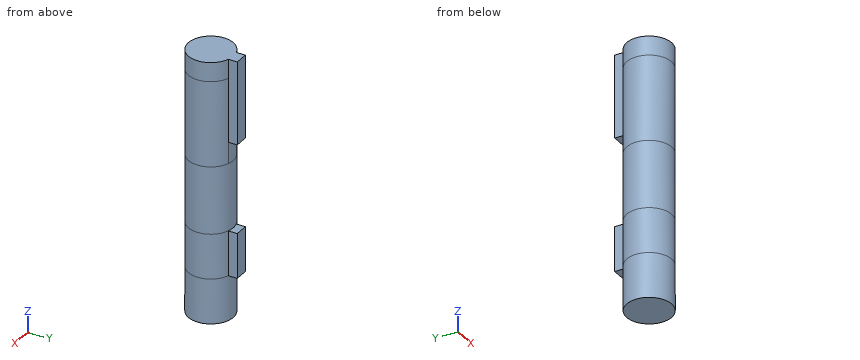
from build123d import *

# Parameters (mm, degrees)
SKETCH1_R            = 5
BOSS_EXTRUDE1_DEPTH  = 20
BOSS_EXTRUDE2_DEPTH  = 10
SKETCH4_R            = 5
BOSS_EXTRUDE3_DEPTH  = 27
BOSS_EXTRUDE4_DEPTH  = 19
SKETCH6_R            = 5
BOSS_EXTRUDE5_DEPTH  = 30
SKETCH7_R            = 5
CUT_EXTRUDE1_DEPTH   = 10
SKETCH8_R            = 6.933887
CUT_EXTRUDE2_DEPTH   = 35
SKETCH9_R            = 5
CUT_EXTRUDE3_DEPTH   = 12
SKETCH10_R           = 5
BOSS_EXTRUDE8_DEPTH  = 15
BOSS_EXTRUDE9_DEPTH  = 10
SKETCH12_R           = 5
BOSS_EXTRUDE10_DEPTH = 10
SKETCH13_R           = 5
CUT_EXTRUDE4_DEPTH   = 28
SKETCH20_R           = 5
CUT_EXTRUDE5_DEPTH   = 2
BOSS_EXTRUDE11_DEPTH = 4.25
CUT_EXTRUDE6_DEPTH   = 22.25
BOSS_EXTRUDE12_DEPTH = 17.5


with BuildPart() as part:
    # Sketch1 → Boss-Extrude1 (new body)
    with BuildSketch(Plane.XY):
        Circle(SKETCH1_R)
    extrude(amount=BOSS_EXTRUDE1_DEPTH)

    # Sketch3 → Boss-Extrude2 (add)
    with BuildSketch(Plane.XY.offset(20)):
        with BuildLine():
            Line((1.5, 6.769696), (-1.5, 6.769696))
            Line((-1.5, 6.769696), (-1.5, 4.769696))
            ThreePointArc((-1.5, 4.769696), (0, -5), (1.5, 4.769696))
            Line((1.5, 4.769696), (1.5, 6.769696))
        make_face()
    extrude(amount=BOSS_EXTRUDE2_DEPTH)

    # Sketch4 → Boss-Extrude3 (add)
    with BuildSketch(Plane.XY.offset(30)):
        Circle(SKETCH4_R)
    extrude(amount=BOSS_EXTRUDE3_DEPTH)

    # Sketch5 → Boss-Extrude4 (add)
    with BuildSketch(Plane.XY.offset(57)):
        with BuildLine():
            Line((-1.5, 4.769696), (-1.5, 6.769696))
            Line((-1.5, 6.769696), (1.5, 6.769696))
            Line((1.5, 6.769696), (1.5, 4.769696))
            ThreePointArc((1.5, 4.769696), (0, -5), (-1.5, 4.769696))
        make_face()
    extrude(amount=BOSS_EXTRUDE4_DEPTH)

    # Sketch6 → Boss-Extrude5 (add)
    with BuildSketch(Plane.XY.offset(76)):
        Circle(SKETCH6_R)
    extrude(amount=BOSS_EXTRUDE5_DEPTH)

    # Sketch7 → Cut-Extrude1 (cut)
    with BuildSketch(Plane(origin=(0, 0, 0), x_dir=(-1, 0, 0), z_dir=(0, 0, -1))):
        Circle(SKETCH7_R)
    extrude(amount=-CUT_EXTRUDE1_DEPTH, mode=Mode.SUBTRACT)

    # Sketch8 → Cut-Extrude2 (cut)
    with BuildSketch(Plane(origin=(0, 0, 10), x_dir=(-1, 0, 0), z_dir=(0, 0, -1))):
        Circle(SKETCH8_R)
    extrude(amount=-CUT_EXTRUDE2_DEPTH, mode=Mode.SUBTRACT)

    # Sketch9 → Cut-Extrude3 (cut)
    with BuildSketch(Plane(origin=(0, 0, 45), x_dir=(-1, 0, 0), z_dir=(0, 0, -1))):
        with Locations(Location((0, 0, 0), (0, 0, 72.542397))):
            Circle(SKETCH9_R)
    extrude(amount=-CUT_EXTRUDE3_DEPTH, mode=Mode.SUBTRACT)

    # Sketch10 → Boss-Extrude8 (add)
    with BuildSketch(Plane(origin=(0, 0, 57), x_dir=(-1, 0, 0), z_dir=(0, 0, -1))):
        Circle(SKETCH10_R)
    extrude(amount=BOSS_EXTRUDE8_DEPTH)

    # Sketch11 → Boss-Extrude9 (add)
    with BuildSketch(Plane(origin=(0, 0, 42), x_dir=(-1, 0, 0), z_dir=(0, 0, -1))):
        with BuildLine():
            Line((-1.5, 6.769696), (1.5, 6.769696))
            Line((1.5, 6.769696), (1.5, 4.769696))
            ThreePointArc((1.5, 4.769696), (0, -5), (-1.5, 4.769696))
            Line((-1.5, 4.769696), (-1.5, 6.769696))
        make_face()
    extrude(amount=BOSS_EXTRUDE9_DEPTH)

    # Sketch12 → Boss-Extrude10 (add)
    with BuildSketch(Plane(origin=(0, 0, 32), x_dir=(-1, 0, 0), z_dir=(0, 0, -1))):
        Circle(SKETCH12_R)
    extrude(amount=BOSS_EXTRUDE10_DEPTH)

    # Sketch13 → Cut-Extrude4 (cut)
    with BuildSketch(Plane.XY.offset(106)):
        with Locations(Location((0, 0, 0), (0, 0, 180))):
            Circle(SKETCH13_R)
    extrude(amount=-CUT_EXTRUDE4_DEPTH, mode=Mode.SUBTRACT)

    # Sketch20 → Cut-Extrude5 (cut)
    with BuildSketch(Plane.XY.offset(78)):
        with Locations(Location((0, 0, 0), (0, 0, 180))):
            Circle(SKETCH20_R)
    extrude(amount=-CUT_EXTRUDE5_DEPTH, mode=Mode.SUBTRACT)

    # Sketch21 → Boss-Extrude11 (add)
    with BuildSketch(Plane.XY.offset(76)):
        with BuildLine():
            Line((1.5, 4.769696), (1.5, 6.769696))
            Line((1.5, 6.769696), (-1.5, 6.769696))
            Line((-1.5, 6.769696), (-1.5, 4.769696))
            ThreePointArc((-1.5, 4.769696), (0, -5), (1.5, 4.769696))
        make_face()
    extrude(amount=BOSS_EXTRUDE11_DEPTH)

    # Sketch22 → Cut-Extrude6 (cut)
    with BuildSketch(Plane(origin=(0, 0, 57), x_dir=(-1, 0, 0), z_dir=(0, 0, -1))):
        with BuildLine():
            Line((1.5, 4.769696), (1.5, 6.769696))
            Line((1.5, 6.769696), (-1.5, 6.769696))
            Line((-1.5, 6.769696), (-1.5, 4.769696))
            ThreePointArc((-1.5, 4.769696), (0, 5), (1.5, 4.769696))
        make_face()
    extrude(amount=-CUT_EXTRUDE6_DEPTH, mode=Mode.SUBTRACT)

    # Sketch23 → Boss-Extrude12 (add)
    with BuildSketch(Plane(origin=(0, 0, 79.25), x_dir=(-1, 0, 0), z_dir=(0, 0, -1))):
        with BuildLine():
            Line((1.5, 4.769696), (1.5, 6.769696))
            Line((1.5, 6.769696), (-1.5, 6.769696))
            Line((-1.5, 6.769696), (-1.5, 4.769696))
            ThreePointArc((-1.5, 4.769696), (0, 5), (1.5, 4.769696))
        make_face()
    extrude(amount=BOSS_EXTRUDE12_DEPTH)


solid = part.part
CAD build for the part. Positions are in the model's coordinates, mm. Round coordinates to 2 decimals unless told otherwise and drop trailing zeros. Write each loop counter-clockwise with the first axis right and the second up, starting at its lowest first coordinate (ties: lowest second). Pieces come first, ordered by that corner, then holes.
(1) Slice it at C-C, the plane y = 2.25. Write the cut outline in (x, z).
(2) Slice it at A-A, the plane y = 5.5. Write the cut outline in (x, z).
(3) Slice it at D-D, the plane z = 58.5. Write the cut outline in (x, y).
(4) Slice it at B-B, the plane x = 0. Write the cut outline in (y, z), and give its area (3 significant figures).
(5) Probe line 1 along X through (y, z) = (5, 71.5); line 2 along X through (y, z) = (3.75, 28); line 3 along Y through (x, z) = (2.75, 49.5). List the from-to ranges inside material, lowest first.
(6) Drop flat-ended pins along their axis: P1, Ø1, axis at x = -0.5, y = 6, coming from the -Z side; P2, Ø0.6, axis at y = 5.5, z = 69, coming from the -X side; P3, Ø2, axis at y = 6, z = 35.5, coming from the +X side. Give the stop position or say it passes through.
From the geometry:
1. outline: (-4.47, 22) - (4.47, 22) - (4.47, 80.25) - (-4.47, 80.25) - close
2. outline: (-1.5, 32) - (1.5, 32) - (1.5, 42) - (-1.5, 42) - close; (-1.5, 61.75) - (1.5, 61.75) - (1.5, 80.25) - (-1.5, 80.25) - close
3. outline: circle Ø10 at (0, 0)
4. outline: (-5, 22) - (5, 22) - (5, 32) - (6.77, 32) - (6.77, 42) - (5, 42) - (5, 61.75) - (6.77, 61.75) - (6.77, 80.25) - (-5, 80.25) - close
4. area: 633 mm2
5. line 1: x = -1.5 to 1.5
5. line 2: x = -3.31 to 3.31
5. line 3: y = -4.18 to 4.18
6. P1: stops at z = 32
6. P2: stops at x = -1.5
6. P3: stops at x = 1.5
